Design review of the part built by this model. Coordinates are the model's own, in mm. A direction names the side the tool comes from. Give positions to 0.01 mm unless a question says otherwise; leave off trailing zeros. Loops run counter-clockwise (first coordinate to the right, second up) from the corner with the lowest first, then second, coordinate; pieces in that order, holes last.
from build123d import *

# Parameters (mm, degrees)
SKETCH1_R           = 14
SKETCH1_R_2         = 2
SKETCH1_R_3         = 7
BOSS_EXTRUDE1_DEPTH = 5
BOSS_EXTRUDE3_START = -5
BOSS_EXTRUDE3_DEPTH = 5
FILLET1_R           = 5
FILLET2_R           = 100


# Some blends are built 0.0001 mm under size
with BuildPart() as part:
    # Sketch1 → Boss-Extrude1 (new body)
    with BuildSketch(Plane(origin=(0, 0, 0), x_dir=(1, 0, 0), z_dir=(0, 1, 0))):
        with Locations(Location((0, 0, 0), (0, 0, 270))):
            Circle(SKETCH1_R)
        with Locations(Location((7.071067812, 7.071067812, 0), (0, 0, 270))):
            Circle(SKETCH1_R_2, mode=Mode.SUBTRACT)
        with Locations(Location((7.071067812, -7.071067812, 0), (0, 0, 270))):
            Circle(SKETCH1_R_2, mode=Mode.SUBTRACT)
        with Locations(Location((-7.071067812, -7.071067812, 0), (0, 0, 270))):
            Circle(SKETCH1_R_2, mode=Mode.SUBTRACT)
        with Locations(Location((-7.071067812, 7.071067812, 0), (0, 0, 270))):
            Circle(SKETCH1_R_2, mode=Mode.SUBTRACT)
        with Locations(Location((0, 0, 0), (0, 0, 270))):
            Circle(SKETCH1_R_3, mode=Mode.SUBTRACT)
    extrude(amount=BOSS_EXTRUDE1_DEPTH)

    # Sketch4 → Boss-Extrude3 (add)
    # profile 1 of 7: a face of its own
    with BuildSketch(Plane(origin=(0, 5, 0), x_dir=(1, 0, 0), z_dir=(0, 1, 0)).offset(BOSS_EXTRUDE3_START)):
        with BuildLine():
            ThreePointArc((-5.711087099, -12.78215491), (-7.937253933, -11.532562595), (-9.899494937, -9.899494937))
            ThreePointArc((-9.899494937, -9.899494937), (-11.532562595, -7.937253933), (-12.78215491, -5.711087099))
            Line((-12.78215491, -5.711087099), (-43.535533906, -36.464466094))
            Line((-43.535533906, -36.464466094), (-36.464466094, -43.535533906))
            Line((-36.464466094, -43.535533906), (-5.711087099, -12.78215491))
        make_face()
        with BuildLine():
            ThreePointArc((-15.541841567, -11.29920088), (-11.29920088, -11.29920088), (-11.29920088, -15.541841567))
            Line((-11.29920088, -15.541841567), (-34.343145751, -38.585786438))
            ThreePointArc((-34.343145751, -38.585786438), (-38.585786438, -38.585786438), (-38.585786438, -34.343145751))
            Line((-38.585786438, -34.343145751), (-15.541841567, -11.29920088))
        make_face(mode=Mode.SUBTRACT)
    # profile 2 of 7: a face of its own
    with BuildSketch(Plane(origin=(0, 5, 0), x_dir=(1, 0, 0), z_dir=(0, 1, 0)).offset(BOSS_EXTRUDE3_START)):
        with BuildLine():
            ThreePointArc((-10.420735139, 9.349239497), (-10.163839474, 9.627895261), (-9.899494937, 9.899494937))
            Line((-9.899494937, 9.899494937), (-11.29920088, 11.29920088))
            ThreePointArc((-11.29920088, 11.29920088), (-13.420521224, 10.420521224), (-15.541841567, 11.29920088))
            Line((-15.541841567, 11.29920088), (-38.585786438, 34.343145751))
            ThreePointArc((-38.585786438, 34.343145751), (-39.464466094, 36.464466094), (-38.585786438, 38.585786438))
            Line((-38.585786438, 38.585786438), (-40, 40))
            Line((-40, 40), (-43.535533906, 36.464466094))
            Line((-43.535533906, 36.464466094), (-13.420521224, 6.349453412))
            Line((-13.420521224, 6.349453412), (-10.420735139, 9.349239497))
        make_face()
    # profile 3 of 7: a face of its own
    with BuildSketch(Plane(origin=(0, 5, 0), x_dir=(1, 0, 0), z_dir=(0, 1, 0)).offset(BOSS_EXTRUDE3_START)):
        with BuildLine():
            ThreePointArc((-12.78215491, 5.711087099), (-11.743192278, 7.622167351), (-10.420735139, 9.349239497))
            Line((-10.420735139, 9.349239497), (-13.420521224, 6.349453412))
            Line((-13.420521224, 6.349453412), (-12.78215491, 5.711087099))
        make_face()
    # profile 4 of 7: a face of its own
    with BuildSketch(Plane(origin=(0, 5, 0), x_dir=(1, 0, 0), z_dir=(0, 1, 0)).offset(BOSS_EXTRUDE3_START)):
        with BuildLine():
            Line((-11.29920088, 11.29920088), (-9.899494937, 9.899494937))
            ThreePointArc((-9.899494937, 9.899494937), (-9.627895261, 10.163839474), (-9.349239497, 10.420735139))
            Line((-9.349239497, 10.420735139), (-6.349453412, 13.420521224))
            Line((-6.349453412, 13.420521224), (-36.464466094, 43.535533906))
            Line((-36.464466094, 43.535533906), (-40, 40))
            Line((-40, 40), (-38.585786438, 38.585786438))
            ThreePointArc((-38.585786438, 38.585786438), (-36.464466094, 39.464466094), (-34.343145751, 38.585786438))
            Line((-34.343145751, 38.585786438), (-11.29920088, 15.541841567))
            ThreePointArc((-11.29920088, 15.541841567), (-10.420521224, 13.420521224), (-11.29920088, 11.29920088))
        make_face()
    # profile 5 of 7: a face of its own
    with BuildSketch(Plane(origin=(0, 5, 0), x_dir=(1, 0, 0), z_dir=(0, 1, 0)).offset(BOSS_EXTRUDE3_START)):
        with BuildLine():
            Line((-6.349453412, 13.420521224), (-9.349239497, 10.420735139))
            ThreePointArc((-9.349239497, 10.420735139), (-7.622167351, 11.743192278), (-5.711087099, 12.78215491))
            Line((-5.711087099, 12.78215491), (-6.349453412, 13.420521224))
        make_face()
    # profile 6 of 7: a face of its own
    with BuildSketch(Plane(origin=(0, 5, 0), x_dir=(1, 0, 0), z_dir=(0, 1, 0)).offset(BOSS_EXTRUDE3_START)):
        with BuildLine():
            ThreePointArc((5.711087099, 12.78215491), (7.937253933, 11.532562595), (9.899494937, 9.899494937))
            ThreePointArc((9.899494937, 9.899494937), (11.532562595, 7.937253933), (12.78215491, 5.711087099))
            Line((12.78215491, 5.711087099), (43.535533906, 36.464466094))
            Line((43.535533906, 36.464466094), (36.464466094, 43.535533906))
            Line((36.464466094, 43.535533906), (5.711087099, 12.78215491))
        make_face()
        with BuildLine():
            ThreePointArc((15.541841567, 11.29920088), (11.29920088, 11.29920088), (11.29920088, 15.541841567))
            Line((11.29920088, 15.541841567), (34.343145751, 38.585786438))
            ThreePointArc((34.343145751, 38.585786438), (38.585786438, 38.585786438), (38.585786438, 34.343145751))
            Line((38.585786438, 34.343145751), (15.541841567, 11.29920088))
        make_face(mode=Mode.SUBTRACT)
    # profile 7 of 7: a face of its own
    with BuildSketch(Plane(origin=(0, 5, 0), x_dir=(1, 0, 0), z_dir=(0, 1, 0)).offset(BOSS_EXTRUDE3_START)):
        with BuildLine():
            ThreePointArc((12.78215491, -5.711087099), (11.532562595, -7.937253933), (9.899494937, -9.899494937))
            ThreePointArc((9.899494937, -9.899494937), (7.937253933, -11.532562595), (5.711087099, -12.78215491))
            Line((5.711087099, -12.78215491), (36.464466094, -43.535533906))
            Line((36.464466094, -43.535533906), (43.535533906, -36.464466094))
            Line((43.535533906, -36.464466094), (12.78215491, -5.711087099))
        make_face()
        with BuildLine():
            ThreePointArc((11.29920088, -15.541841567), (11.29920088, -11.29920088), (15.541841567, -11.29920088))
            Line((15.541841567, -11.29920088), (38.585786438, -34.343145751))
            ThreePointArc((38.585786438, -34.343145751), (38.585786438, -38.585786438), (34.343145751, -38.585786438))
            Line((34.343145751, -38.585786438), (11.29920088, -15.541841567))
        make_face(mode=Mode.SUBTRACT)
    extrude(amount=BOSS_EXTRUDE3_DEPTH)

    # Fillet1
    fillet1_edges = [part.edges().sort_by_distance(p)[0] for p in [
        (-36.464466094, 2.5, 43.535533906),
        (-43.535533906, 2.5, 36.464466094),
        (-43.535533906, 2.5, -36.464466094),
        (-36.464466094, 2.5, -43.535533906),
        (36.464466094, 2.5, -43.535533906),
        (43.535533906, 2.5, -36.464466094),
        (36.464466094, 2.5, 43.535533906),
        (43.535533906, 2.5, 36.464466094),
    ]]
    fillet(fillet1_edges, radius=FILLET1_R - 0.0001)  # a hair under: the kernel refuses the full size

    # Fillet2
    # the kernel refuses this fillet: 100 mm, written as the material it adds along each edge
    with BuildSketch(Plane(origin=(-5.711087099, 0, 12.78215491), x_dir=(0.9998484998051017, 0, 0.017406247082228966), z_dir=(0, 1, 0)), Plane(origin=(-12.78215491, 0, -5.711087099), x_dir=(-0.017406247082221098, 0, 0.9998484998051018), z_dir=(0, 1, 0))) as fillet2_piece_1:
        with BuildLine():
            CenterArc((50.173554479, -91.997335747), FILLET2_R, 113.07781271, 22.919542152)
            Line((-21.757218493, -22.528177844), (0, 0))
            ThreePointArc((0, 0), (5.487732521, -1.120372995), (10.975465042, 0))
        make_face()
    extrude(amount=5)
    with BuildSketch(Plane(origin=(5.711087099, 0, 12.78215491), x_dir=(0.7071067811865421, 0, 0.7071067811865529), z_dir=(0, 1, 0)), Plane(origin=(-12.78215491, 0, 5.711087099), x_dir=(-0.7071067811865551, 0, 0.7071067811865399), z_dir=(0, 1, 0))) as fillet2_piece_2:
        with BuildLine():
            CenterArc((31.31924893, -100), FILLET2_R, 90, 22.919542152)
            ThreePointArc((-7.624563141, -7.894736842), (-3.006388615, -4.725682106), (0, 0))
            Line((0, 0), (31.31924893, 0))
        make_face()
    extrude(amount=5)
    with BuildSketch(Plane(origin=(12.78215491, 0, 5.711087099), x_dir=(0.7071067811865436, 0, 0.7071067811865516), z_dir=(0, 1, 0)), Plane(origin=(5.711087099, 0, -12.78215491), x_dir=(0.7071067811865498, 0, -0.7071067811865454), z_dir=(0, 1, 0))) as fillet2_piece_3:
        with BuildLine():
            CenterArc((31.31924893, 100), FILLET2_R, 247.080457848, 22.919542152)
            ThreePointArc((-7.624563141, 7.894736842), (-3.006388615, 4.725682106), (0, 0))
            Line((0, 0), (31.31924893, 0))
        make_face()
    extrude(amount=5)
    with BuildSketch(Plane(origin=(12.78215491, 0, -5.711087099), x_dir=(0.01740624708221406, 0, 0.9998484998051019), z_dir=(0, 1, 0)), Plane(origin=(-5.711087099, 0, -12.78215491), x_dir=(0.9998484998051018, 0, -0.017406247082221094), z_dir=(0, 1, 0))) as fillet2_piece_4:
        with BuildLine():
            CenterArc((50.173554479, 91.997335747), FILLET2_R, 224.002645138, 22.919542152)
            Line((-21.757218493, 22.528177844), (0, 0))
            ThreePointArc((0, 0), (5.487732521, 1.120372995), (10.975465042, 0))
        make_face()
    extrude(amount=5)


solid = part.part
Q1. Take a section at C-C (y = 3.5). Give the number of separate pieces and of enclosed holes in the cut face, plus the area to 3 significant figures.
Results:
separate pieces: 1
enclosed holes: 9
area: 1,670 mm2
Q2. Tool access review of faces 1 (the face through (-24.05, 2.46, 14.97)), 2 (the face through (22.982, 2.465, 27.225)), 3 (the face through (30.43, 2.46, -37.5)): name each direction out of +Z, -Z, +X, -X, +Y, -Y from which nothing blocks a thin tool from reaching the whole face with its end or side.
Results:
face 1: -X, +Y, -Y
face 2: +Y, -Y
face 3: -Z, +Y, -Y
Q3. Take a section at B-B (x = -1). Give the boundary of the cut face in (y, z), plus the area to 3 significant figures.
Results:
outline: (0, -15.77) - (5, -15.77) - (5, -6.93) - (0, -6.93) - close; (0, 6.93) - (5, 6.93) - (5, 15.77) - (0, 15.77) - close
area: 88.4 mm2
Q4. Draft analysis for pull direction X (two halves, no side actions). For faces 4 (the face through (-22.982, 2.465, -27.225)), 5 (the face through (41.464, 2.535, 36.409)), 6 (the face through (38.54, 2.46, -38.63)), 7 (the face through (-37.43, 2.46, 30.36)), state which applies: pulls with the +X half, pulls with the -X half, needs draft (parallel to the pull), parting line crosses it, or undercut.
Results:
face 4: undercut
face 5: pulls with the +X half
face 6: undercut
face 7: pulls with the -X half
Q5. Take a section at A-A (z = 24). Give the boundary of the cut face in (x, y).
Results:
outline: (-31.27, 0) - (-28.24, 0) - (-28.24, 5) - (-31.27, 5) - close; (-19.76, 0) - (-14.9, 0) - (-14.9, 5) - (-19.76, 5) - close; (14.9, 0) - (19.76, 0) - (19.76, 5) - (14.9, 5) - close; (28.24, 0) - (31.27, 0) - (31.27, 5) - (28.24, 5) - close
Q6. Insertion check: pin 1 (1 mm diameter, centred on x = -12.5, y = 4.5, fed in from -Z); pin 2 (3 mm diameter, centred on x = 7.07, z = -7.07, fed in from +Y). Each pin has a flat end and moves straight along its axis. Give the tip position at first contact, or say it passes through.
Results:
pin 1: stops at z = -22.69
pin 2: passes through
Q7. Wall thickness on line 1 (X direction, y = 3.1, z = 35.5); line 2 (X direction, y = 3.85, z = 15.5); line 3 (Z direction, x = -32.5, y = 3.6): over which ranges is each line inside the solid? List them lowest first.
Results:
line 1: x = -41.37 to -39.31, -31.26 to -28.43, 28.43 to 31.26, 39.31 to 41.37
line 2: x = -24.43 to -19.74, -11.26 to -0.45, 0.45 to 11.26, 19.74 to 24.43
line 3: z = -39.57 to -36.74, -28.26 to -25.34, 25.34 to 28.26, 36.74 to 39.57
